from build123d import *

# Parameters (mm, degrees)
BOSS_EXTRUDE1_DEPTH = 30
BOSS_EXTRUDE2_DEPTH = 30
SKETCH3_R           = 1.5
BOSS_EXTRUDE3_DEPTH = 30
SKETCH4_R           = 1.100328426
BOSS_EXTRUDE4_DEPTH = 0.1
SKETCH5_W           = 14
SKETCH5_H           = 24
SKETCH5_W_2         = 19
CUT_EXTRUDE1_DEPTH  = 6.1
FILLET1_R           = 2
FILLET2_R           = 1
FILLET3_R           = 5
FILLET4_R           = 1


with BuildPart() as part:
    # Sketch1 → Boss-Extrude1 (new body)
    with BuildSketch(Plane(origin=(0, 0, 0), x_dir=(1, 0, 0), z_dir=(0, 1, 0))):
        Polygon((0, 0), (-80, 0), (0, 200), align=None)
        Polygon((-5, 10), (-70.614835193, 10), (-5, 174.037087982), align=None, mode=Mode.SUBTRACT)
    extrude(amount=BOSS_EXTRUDE1_DEPTH)

    # Sketch2 → Boss-Extrude2 (add)
    with BuildSketch(Plane(origin=(0, 0, 0), x_dir=(1, 0, 0), z_dir=(0, 1, 0))):
        Polygon((-5, 35), (-60.614835193, 35), (-59.814835193, 37), (-5, 37), align=None)
        Polygon((-51.014835193, 59), (-51.814835193, 57), (-5, 57), (-5, 59), align=None)
        Polygon((-43.014835193, 79), (-5, 79), (-5, 81), (-42.214835193, 81), align=None)
        Polygon((-34.214835193, 101), (-33.414835193, 103), (-5, 103), (-5, 101), align=None)
        Polygon((-21.414835193, 133), (-21.014835193, 134), (-5, 134), (-5, 133), align=None)
        Polygon((-9.014835193, 164), (-8.614835193, 165), (-5, 165), (-5, 164), align=None)
    extrude(amount=BOSS_EXTRUDE2_DEPTH)

    # Sketch3 → Boss-Extrude3 (add)
    with BuildSketch(Plane(origin=(0, 0, 0), x_dir=(1, 0, 0), z_dir=(0, 1, 0))):
        Polygon((-2, 0), (-2, -5), (0, -5), (0, -7), (-10, -7), (-10, -5), (-8, -5), (-8, 0), align=None)
        with BuildLine():
            Line((-80, 0), (-81.034384241, -2.585960604))
            ThreePointArc((-81.034384241, -2.585960604), (-76.228484638, -11.382716514), (-68.499285751, -5))
            ThreePointArc((-68.499285751, -5), (-67.034819657, -1.464466094), (-63.499285751, 0))
            Line((-63.499285751, 0), (-80, 0))
        make_face()
        with Locations((-74.999285751, -5)):
            Circle(SKETCH3_R, mode=Mode.SUBTRACT)
    extrude(amount=BOSS_EXTRUDE3_DEPTH)

    # Sketch4 → Boss-Extrude4 (add)
    with BuildSketch(Plane(origin=(0, 0, 0), x_dir=(0, 0, -1), z_dir=(1, 0, 0))):
        with Locations((144.319162345, 14.586186638)):
            Circle(SKETCH4_R)
    extrude(amount=BOSS_EXTRUDE4_DEPTH)

    # Sketch5 → Cut-Extrude1 (cut, through all)
    with BuildSketch(Plane.ZY.offset(5)):
        with Locations((-91, 15)):
            Rectangle(SKETCH5_W, SKETCH5_H)
        with Locations((-69, 15)):
            Rectangle(SKETCH5_W, SKETCH5_H)
        with Locations((-47, 15)):
            Rectangle(SKETCH5_W, SKETCH5_H)
        with Locations((-22.5, 15)):
            Rectangle(SKETCH5_W_2, SKETCH5_H)
    extrude(amount=-CUT_EXTRUDE1_DEPTH, mode=Mode.SUBTRACT)

    # Fillet1
    fillet1_edges = [part.edges().sort_by_distance(p)[0] for p in [
        (-5, 15, -10),
        (-70.614835193, 15, -10),
        (-60.614835193, 15, -35),
        (-59.814835193, 15, -37),
        (-5, 15, -37),
        (-5, 15, -35),
        (-5, 15, -57),
        (-51.814835193, 15, -57),
        (-51.014835193, 15, -59),
        (-5, 15, -59),
        (-5, 15, -81),
        (-5, 15, -79),
        (-43.014835193, 15, -79),
        (-42.214835193, 15, -81),
        (-33.414835193, 15, -103),
        (-5, 15, -103),
        (-5, 15, -101),
        (-34.214835193, 15, -101),
        (-21.014835193, 15, -134),
        (-5, 15, -134),
        (-5, 15, -133),
        (-21.414835193, 15, -133),
        (-5, 15, -164),
        (-9.014835193, 15, -164),
    ]]
    fillet(fillet1_edges, radius=FILLET1_R)

    # Fillet2
    fillet2_edges = [part.edges().sort_by_distance(p)[0] for p in [
        (-5, 15, -174.037087982),
        (-8.614835193, 15, -165),
        (-5, 15, -165),
    ]]
    fillet(fillet2_edges, radius=FILLET2_R)

    # Fillet3
    fillet3_edges = [part.edges().sort_by_distance(p)[0] for p in [
        (-2.5, 27, -84),
        (-2.5, 3, -84),
        (-2.5, 3, -98),
        (-2.5, 27, -98),
        (-2.5, 27, -62),
        (-2.5, 3, -62),
        (-2.5, 3, -76),
        (-2.5, 27, -76),
        (-2.5, 27, -40),
        (-2.5, 3, -40),
        (-2.5, 3, -54),
        (-2.5, 27, -54),
        (-2.5, 27, -13),
        (-2.5, 3, -13),
        (-2.5, 3, -32),
        (-2.5, 27, -32),
    ]]
    fillet(fillet3_edges, radius=FILLET3_R)

    # Fillet4
    fillet4_edges = [part.edges().sort_by_distance(p)[0] for p in [
        (0, 30, 6),
        (0, 0, 6),
        (-10, 30, 6),
        (-10, 0, 6),
    ]]
    fillet(fillet4_edges, radius=FILLET4_R)


solid = part.part
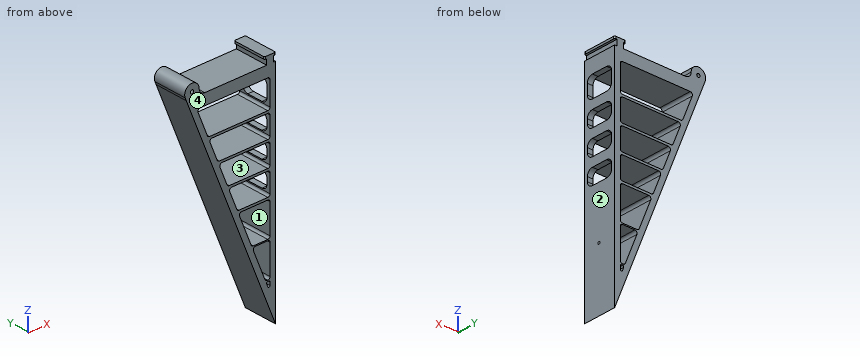
Read the model definition and answer for the solid it produces. Units are mm, in the model's axes. Face numbers are marked on the shaded views. Round coordinates to 2 decimals unless told otherwise and drop trailing zeros. Write each loop counter-clockwise with the first axis right and the second up, starting at its lowest first coordinate (ties: lowest second). Pieces come first, ordered by that corner, then holes. Notation, with made-up numbers: M 21.5,19 L 52.5,19 A16 ccw 52.5,45 Z; hole C 41,1.25 d6. An arc over 180 degrees is marked long. Use a Markdown table: item, result.
1) The part is cut by section A-A (x = -26). Write down the section's boundary in (y, z).
Answers follow:
| item | result |
|---|---|
| outline | M 0,-135 L 30,-135 L 30,-121.54 L 0,-121.54 Z; M 0,-103 L 30,-103 L 30,-101 L 0,-101 Z; M 0,-81 L 30,-81 L 30,-79 L 0,-79 Z; M 0,-59 L 30,-59 L 30,-57 L 0,-57 Z; M 0,-37 L 30,-37 L 30,-35 L 0,-35 Z; M 0,-10 L 30,-10 L 30,0 L 0,0 Z |
2) Flat-ended cylindrical pins translate along their axes: pin 1 (1 mm diameter, centred on x = -40.5, y = 25, fed in from +Z); pin 2 (4 mm diameter, centred on y = 24, z = -172.5, fed in from +X); pin 3 (1 mm diameter, centred on x = -1, y = 20, fed in from +Z). Find the tip coordinate at first contact, or state that the pin passes through.
Answers follow:
| item | result |
|---|---|
| pin 1 | stops at z = 0 |
| pin 2 | stops at x = 0 |
| pin 3 | stops at z = 7 |
3) Straight lines are drawn through the part: line 1 along X through (y, z) = (4.75, -83.5); line 2 along X through (y, z) = (21.75, -124); line 3 along X through (y, z) = (14, -35.5). For each, find the intervals that lie inside material, in ascending order. Write a range as [from, to].
Answers follow:
| item | result |
|---|---|
| line 1 | x = [-46.6, -41.2], [-5, 0] |
| line 2 | x = [-30.4, -25.01], [-5, 0] |
| line 3 | x = [-65.8, 0] |
4) For a pull along X with two mould halves and no side action, classify the marked faces 1, 2, 3 and 4 as pulls with the +X half, pulls with the -X half, needs draft (parallel to the pull), parting line crosses it, or undercut.
Answers follow:
| item | result |
|---|---|
| face 1 | undercut |
| face 2 | pulls with the +X half |
| face 3 | undercut |
| face 4 | needs draft |
5) The part is cut by section B-B (y = 11.25). Give the number of separate pieces and of enclosed holes in the cut face, plus the area to 3 significant figures.
Answers follow:
| item | result |
|---|---|
| separate pieces | 1 |
| enclosed holes | 4 |
| area | 2,880 mm2 |
